from build123d import *

# Parameters (mm, degrees)
F1_DEPTH    = 3.175
F2_W        = 9.525
F2_H        = 1.4478
F3_DEPTH    = 25.4
F4_R        = 15.842845787
F4_R_2      = 3.2177044056
F4_R_3      = 1.5904309239
F5_DEPTH    = 1.27
F6_T1_DEPTH = 31.75
F6_T3_DEPTH = 27.3506510316
F7_R        = 1.27
F9_DEPTH    = 25.4


# Not quite as in the source:
# - a fillet or chamfer that OpenCascade refuses, or shapes differently, is made with other operations: its cross-section is extruded or revolved along the edge and cut away or added


with BuildPart() as f1:
    # F0 (on Top) → F1 (new body, symmetric)
    with BuildSketch(Plane.XY):
        Polygon((17.7787664203, 21.9838270611), (-17.1462335797, 21.9838270611), (-17.1462335797, -12.9411729389), (-14.9237335797, -12.9411729389), (-14.9237335797, -28.8161729389), (-3.4937335797, -28.8161729389), (-3.4937335797, -12.9411729389), (4.1262664203, -12.9411729389), (4.1262664203, -28.8161729389), (15.5562664203, -28.8161729389), (15.5562664203, -12.9411729389), (17.7787664203, -12.9411729389), align=None)
    extrude(amount=F1_DEPTH, both=True)

    # F2 (on Right) → F3 (cut, symmetric)
    with BuildSketch(Plane.YZ):
        with Locations((-19.2911729389, -2.4511)):
            Rectangle(F2_W, F2_H)
        with Locations((-19.2911729389, 2.4511)):
            Rectangle(F2_W, F2_H)
    extrude(amount=F3_DEPTH, both=True, mode=Mode.SUBTRACT)

    # F4 (on face) → F5 (cut)
    with BuildSketch(Plane.XY.offset(3.175)):
        with Locations((0.4921501707, 3.9010436143)):
            Circle(F4_R)
        with BuildLine():
            Line((-2.1375703251, 6.8868143019), (0.4050256131, 11.0911789057))
            ThreePointArc((0.4050256131, 11.0911789057), (0.3466666466, 8.3599053372), (1.5539010716, 5.9092225511))
            ThreePointArc((1.5539010716, 5.9092225511), (-0.0735190255, 1.7484484648), (3.4811131017, -0.9580488308))
            Line((3.4811131017, -0.9580488308), (-4.5523895124, -4.9100595401))
            Line((-4.5523895124, -4.9100595401), (-2.4823771265, -1.3211422242))
            Line((-2.4823771265, -1.3211422242), (-9.0284545614, -5.1116843583))
            Line((-9.0284545614, -5.1116843583), (-4.7554110557, 1.9540993141))
            Line((-4.7554110557, 1.9540993141), (-7.5469899631, 0.4189560082))
            Line((-7.5469899631, 0.4189560082), (-4.8280507742, 5.1179121089))
            ThreePointArc((-4.8280507742, 5.1179121089), (-1.9693373897, 3.7003874584), (-2.1375703251, 6.8868143019))
        make_face(mode=Mode.SUBTRACT)
        with Locations((3.4971262654, 2.7505044746)):
            Circle(F4_R_2, mode=Mode.SUBTRACT)
        with Locations((-2.9845039712, 5.2444444735)):
            Circle(F4_R_3, mode=Mode.SUBTRACT)
        with BuildLine():
            ThreePointArc((2.1821519983, 6.218135758), (7.6895432258, 14.3852639145), (6.7216994367, 4.5823756229))
            ThreePointArc((6.7216994367, 4.5823756229), (4.7543334077, 6.2394949077), (2.1821519983, 6.218135758))
        make_face(mode=Mode.SUBTRACT)
    extrude(amount=-F5_DEPTH, mode=Mode.SUBTRACT)

    # F6: fillet of radius 5.08 on 4 edges, made by hand

    # F6_s2 → F6_t1 (cut)
    with BuildSketch(Plane.XY.offset(-15.875)):
        with BuildLine():
            ThreePointArc((17.7787664203, 16.9038270611), (16.2908688687, 20.4959295096), (12.6987664203, 21.9838270611))
            Line((12.6987664203, 21.9838270611), (17.7787664203, 21.9838270611))
            Line((17.7787664203, 21.9838270611), (17.7787664203, 16.9038270611))
        make_face()
        with BuildLine():
            ThreePointArc((-12.0662335797, 21.9838270611), (-15.6583360282, 20.4959295096), (-17.1462335797, 16.9038270611))
            Line((-17.1462335797, 16.9038270611), (-17.1462335797, 21.9838270611))
            Line((-17.1462335797, 21.9838270611), (-12.0662335797, 21.9838270611))
        make_face()
    extrude(amount=F6_T1_DEPTH, mode=Mode.SUBTRACT)

    # F6_s4 → F6_t3 (cut)
    with BuildSketch(Plane.XY.offset(-13.6753255158)):
        with BuildLine():
            ThreePointArc((-14.9237335797, -12.9411729388), (-16.5563616403, -11.1169951731), (-17.1462335797, -8.7410427325))
            Line((-17.1462335797, -8.7410427325), (-17.1462335797, -12.9411729389))
            Line((-17.1462335797, -12.9411729389), (-14.9237335797, -12.9411729388))
        make_face()
        with BuildLine():
            ThreePointArc((17.7787664203, -8.7410427325), (17.1888944808, -11.1169951731), (15.5562664203, -12.9411729388))
            Line((15.5562664203, -12.9411729388), (17.7787664203, -12.9411729389))
            Line((17.7787664203, -12.9411729389), (17.7787664203, -8.7410427325))
        make_face()
    extrude(amount=F6_T3_DEPTH, mode=Mode.SUBTRACT)

    # F7
    f7_edges = [f1.edges().sort_by_distance(p)[0] for p in [
        (-14.923734, -14.528673, 2.4511),
        (-3.493734, -14.528673, 2.4511),
        (15.556266, -14.528673, 2.4511),
        (4.126266, -14.528673, 2.4511),
        (15.556266, -14.528673, -2.4511),
        (4.126266, -14.528673, -2.4511),
        (-14.923734, -14.528673, -2.4511),
        (-3.493734, -14.528673, -2.4511),
        (-3.493734, -24.053673, -2.4511),
        (-3.493734, -24.053673, 2.4511),
        (15.556266, -24.053673, -2.4511),
        (15.556266, -24.053673, 2.4511),
        (15.556266, -28.816173, 0),
        (4.126266, -28.816173, 0),
        (-3.493734, -28.816173, 0),
        (-14.923734, -28.816173, 0),
        (-14.923734, -24.053673, 2.4511),
        (-14.923734, -24.053673, -2.4511),
        (4.126266, -24.053673, 2.4511),
        (4.126266, -24.053673, -2.4511),
    ]]
    fillet(f7_edges, radius=F7_R)

    # F8 (on face) → F9 (cut)
    with BuildSketch(Plane.XY.offset(3.175)):
        with BuildLine():
            ThreePointArc((-17.1462335797, 16.9038270611), (-15.6583360282, 20.4959295096), (-12.0662335797, 21.9838270611))
            Line((-12.0662335797, 21.9838270611), (-17.1462335797, 21.9838270611))
            Line((-17.1462335797, 21.9838270611), (-17.1462335797, 16.9038270611))
        make_face()
        with BuildLine():
            ThreePointArc((12.6987664203, 21.9838270611), (16.2908688687, 20.4959295095), (17.7787664203, 16.9038270611))
            Line((17.7787664203, 16.9038270611), (17.7787664203, 21.9838270611))
            Line((17.7787664203, 21.9838270611), (12.6987664203, 21.9838270611))
        make_face()
        with BuildLine():
            ThreePointArc((0.3162664203, 21.9838270611), (12.6641185867, 16.8691792276), (17.7787664203, 4.5213270611))
            Line((17.7787664203, 4.5213270611), (17.7787664203, 16.9038270611))
            ThreePointArc((17.7787664203, 16.9038270611), (16.2908688687, 20.4959295095), (12.6987664203, 21.9838270611))
            Line((12.6987664203, 21.9838270611), (0.3162664203, 21.9838270611))
        make_face()
        with BuildLine():
            ThreePointArc((-17.1462335797, 4.5213270326), (-12.0315857563, 16.8691792175), (0.3162664203, 21.9838270611))
            Line((0.3162664203, 21.9838270611), (-12.0662335797, 21.9838270611))
            ThreePointArc((-12.0662335797, 21.9838270611), (-15.6583360282, 20.4959295096), (-17.1462335797, 16.9038270611))
            Line((-17.1462335797, 16.9038270611), (-17.1462335797, 4.5213270326))
        make_face()
    extrude(amount=-F9_DEPTH, mode=Mode.SUBTRACT)


solid = f1.part
Read the model definition and answer for the solid it produces. Units are mm, in the model's axes. A direction names the side the tool comes from. Give positions to 0.01 mm unless a question says otherwise; leave off trailing zeros. Write each loop counter-clockwise with the first axis right and the second up, starting at its lowest first coordinate (ties: lowest second). Pieces come first, ordered by that corner, then holes. Notation, with made-up numbers: (63.5, -23.5) - (72.5, -23.5) arc R25 ccw to (72.5, -5.5) - close; hole circle Ø10 at (58, 63.5). An arc over 180 degrees is marked (long way). Answer in a Markdown table with one row per item. Add a question column.
Item 1: Section B-B, the plane z = -2.5 is taken. Count the separate pieces of the cut face and the enclosed holes in it, and give its area (3 significant figures).
Item 2: Section A-A, the plane y = -22 is taken. Write down the section's boundary in (x, z).
Item 3: Find the intervals of material crossed by L1, parallel to Y at x = -8, z = 2.25; L2, parallel to X at y = -16.5, z = 0; L3, parallel to X at y = 1, z = 2.75, in increasing order.
Item 4: Determine the mould class of faces 1 (the face through (-9, -26, -3.175)), 2 (the face through (10, -19, 1.727)), 3 (the face through (4.488, -28.434, 0.044)) for opening direction Y: pulls with the +Y half, pulls with the -Y half, needs draft (parallel to the pull), parting line crosses it, or undercut.
Item 5: A tool of negligible diameter and unlimited length cuts with its end or side. For faces 4 (the face through (0.338, 8.398, 2.549)), 5 (the face through (-9, -24.054, -2)), 6 (the face through (15.194, -24.436, -2.461)), from which of +Z, -Z, +X, -X, +Y, -Y can it reach the whole face along a straight path? Write none if from no direction.
Item 6: Flat-ended cylindrical pins translate along their axes: P1, Ø1, axis at y = 5.5, z = 2, coming from the +X side; P2, Ø1.2, axis at x = -11, z = -2.5, coming from the +Y side; P3, Ø1, axis at x = 3, y = -6.5, coming from the +Z side (3 decimals). Find the tip coordinate at first contact, or state that the pin passes through.
Item 7: Section C-C, the plane x = -13 is taken. Write down the section's boundary in (y, z) (3 decimals), and give its area (3 significant figures).
Recorded:
| question | item | result |
|---|---|---|
| 1 | separate pieces | 3 |
| 1 | enclosed holes | 0 |
| 1 | area | 1,220 mm2 |
| 2 | outline | (-14.92, -1.73) - (-3.49, -1.73) - (-3.49, 1.73) - (-14.92, 1.73) - close; (4.13, -1.73) - (15.56, -1.73) - (15.56, 1.73) - (4.13, 1.73) - close |
| 3 | L1 | y = -28.82 to -24.05, -14.53 to -9.47, -4.52 to -3.41, 17.28 to 19.88 |
| 3 | L2 | x = -14.92 to -3.49, 4.13 to 15.56 |
| 3 | L3 | x = -17.15 to -15.08, -7.21 to -6.49, -5.33 to 0.23, 0.8 to 6.2, 16.07 to 17.78 |
| 4 | face 1 | needs draft |
| 4 | face 2 | undercut |
| 4 | face 3 | pulls with the -Y half |
| 5 | face 4 | +Z |
| 5 | face 5 | -Z, +X, -X |
| 5 | face 6 | -Z, +X |
| 6 | P1 | stops at x = 17.77 |
| 6 | P2 | stops at y = 18.31 |
| 6 | P3 | stops at z = 1.905 |
| 7 | outline | (-28.816, -3.175) - (-24.054, -3.175) - (-24.054, -1.727) - (-14.529, -1.727) - (-14.529, -3.175) - (15.818, -3.175) - (15.818, 3.175) - (12.205, 3.175) - (12.205, 1.905) - (-4.403, 1.905) - (-4.403, 3.175) - (-14.529, 3.175) - (-14.529, 1.727) - (-24.054, 1.727) - (-24.054, 3.175) - (-28.816, 3.175) - close |
| 7 | area | 235 mm2 |
